The listing builds one solid part. Answer for the finished solid, in the listing's coordinates (mm). A direction names the side the tool comes from. Coordinates: 2 decimals unless noted, no trailing zeros. Order: outer loops, then holes, each group sorted by start corner. A loop starts at its lowest first (then second) coordinate and runs counter-clockwise, first axis right, second up. Notation, with made-up numbers: (45.25, -6) -> (55.25, -6) arc R24 ccw to (55.25, 27) -> close; hole circle Ø6 at (35, 81.5). An arc over 180 degrees is marked (long way). Write each question's results on one line, items separated by ' | '. Start each with the question number.
(1) A tool of negligible diameter and unlimited length cuts with its end or side. For faces 1 (the face through (125, -2, 9.7)), 2 (the face through (273.001, -1.959, 6.783)), 3 (the face through (157, -2, 0)), from which of +Z, -Z, +X, -X, +Y, -Y can it reach the whole face along a straight path? Write none if from no direction.
(2) Determine the mould class of faces 4 (the face through (-22.41, -1.96, 8.88)), 5 (the face through (155, -2, 3)), 6 (the face through (126, 10.564, 11)), 7 (the face through (70.778, -1.959, 3.397)) for opening direction Z: +Z half, -Z half, draft (parallel to the pull), parting line (faces both ways), or undercut.
(3) The part is cut by section A-A, the plane x = 162. Give the vertices of the cut face in (y, z), then the cut area to 3 significant figures.
(4) Straight lines are drawn through the part: L1, parallel to Z at x = 164.5, y = 3.5; L2, parallel to Z at x = 54, y = -12.25; L3, parallel to Z at x = 231, y = -4.75. For each, find the intervals that lie inside material, in ascending order.
(5) The part is cut by section C-C, the plane x = 42. Give the vertices of the cut face in (y, z), then the cut area to 3 significant figures.
(6) The part is cut by section D-D, the plane x = 237. Give the vertices of the cut face in (y, z).
(7) Given pin 1 (12 mm diameter, centred on x = 184.5, y = -3.5, fed in from -Z); pin 2 (1.5 mm diameter, centred on x = 195.5, y = 6.5, fed in from -Z); pin 3 (3 mm diameter, centred on x = 97.47, y = 5.36, fed in from -Z), each flat-ended and moving along its own axis, determine where each tip first touches the part or whether it passes through.
```python
from build123d import *

# Parameters (mm, degrees)
SKETCH1_W                 = 304.8
SKETCH1_H                 = 25.4
BOSS_EXTRUDE2_DEPTH       = 12.7
FILLET1_R                 = 12.7
CUT_EXTRUDE3_DEPTH        = 281.209703849
SKETCH8_W                 = 70
SKETCH8_H                 = 25.4
BOSS_EXTRUDE3_DEPTH       = 9.7
CUT_EXTRUDE4_DEPTH        = 281.209703849
CUT_EXTRUDE5_DEPTH        = 281.209703849
F_6_CLEARANCE_HOLE1_D     = 3.7973
F_6_CLEARANCE_HOLE1_DEPTH = 3


with BuildPart() as part:
    # Sketch1 → Boss-Extrude2 (new body)
    with BuildSketch(Plane.XY):
        with Locations((126.366978193, -2.136448598)):
            Rectangle(SKETCH1_W, SKETCH1_H)
    extrude(amount=BOSS_EXTRUDE2_DEPTH)

    # Fillet1
    fillet1_edges = [part.edges().sort_by_distance(p)[0] for p in [
        (-26.033021807, -2.136448598, 12.7),
        (278.766978193, -2.136448598, 12.7),
    ]]
    fillet(fillet1_edges, radius=FILLET1_R - 0.0001)  # a hair under: the kernel refuses the full size

    # Sketch6 → Cut-Extrude3 (cut, through all)
    with BuildSketch(Plane(origin=(0, 10.563551402, 0), x_dir=(1, 0, 0), z_dir=(0, 1, 0))):
        with BuildLine():
            Line((-23.033021807, 0), (275.766978193, 0))
            ThreePointArc((275.766978193, 0), (272.925913971, -6.858935778), (266.066978193, -9.7))
            Line((266.066978193, -9.7), (-13.333021807, -9.7))
            ThreePointArc((-13.333021807, -9.7), (-20.191957584, -6.858935778), (-23.033021807, 0))
        make_face()
    extrude(amount=-CUT_EXTRUDE3_DEPTH, mode=Mode.SUBTRACT)

    # Sketch8 → Boss-Extrude3 (add)
    with BuildSketch(Plane(origin=(0, 0, 9.7), x_dir=(-1, 0, 0), z_dir=(0, 0, -1))):
        with Locations((-180.266978193, -2.136448598)):
            Rectangle(SKETCH8_W, SKETCH8_H)
        with Locations((-72.466978193, -2.136448598)):
            Rectangle(SKETCH8_W, SKETCH8_H)
    extrude(amount=BOSS_EXTRUDE3_DEPTH)

    # Sketch9 → Cut-Extrude4 (cut, through all)
    with BuildSketch(Plane(origin=(0, 10.563551402, 0), x_dir=(1, 0, 0), z_dir=(0, 1, 0))):
        Polygon((145.266978193, -9.7), (165.266978193, -9.7), (192.266978193, -9.7), (165.266978193, -3), (145.266978193, -3), align=None)
        Polygon((215.266978193, -6.7), (195.266978193, -6.7), (168.266978193, 0), (215.266978193, 0), align=None)
    extrude(amount=-CUT_EXTRUDE4_DEPTH, mode=Mode.SUBTRACT)

    # Sketch12 → Cut-Extrude5 (cut, through all)
    with BuildSketch(Plane(origin=(0, 10.563551402, 0), x_dir=(1, 0, 0), z_dir=(0, 1, 0))):
        Polygon((107.466978193, -9.7), (107.466978193, -3), (87.466978193, -3), (60.466978193, -9.7), align=None)
        Polygon((37.466978193, -6.7), (57.466978193, -6.7), (84.466978193, 0), (37.466978193, 0), align=None)
    extrude(amount=-CUT_EXTRUDE5_DEPTH, mode=Mode.SUBTRACT)

    # #6 Clearance Hole1
    with Locations(Plane.XY.offset(3)):
        with Locations((97.466978193, 5.363551402), (155.266978193, 5.363551402), (155.266978193, -9.636448598), (97.466978193, -9.636448598)):
            Hole(F_6_CLEARANCE_HOLE1_D / 2, depth=F_6_CLEARANCE_HOLE1_DEPTH)


solid = part.part
```
Established:
1) face 1: +Y, -Y | face 2: -Z, +Y, -Y | face 3: -Z, +X, -X, +Y, -Y
2) face 4: +Z half | face 5: undercut | face 6: draft | face 7: -Z half
3) outline: (-14.84, 0) -> (10.56, 0) -> (10.56, 3) -> (-14.84, 3) -> close; (-14.84, 9.7) -> (10.56, 9.7) -> (10.56, 12.7) -> (-14.84, 12.7) -> close | area: 152 mm^2
4) L1: z = 0 to 3, 9.7 to 12.7 | L2: z = 6.7 to 12.7 | L3: z = 9.7 to 12.7
5) outline: (-14.84, 6.7) -> (10.56, 6.7) -> (10.56, 12.7) -> (-14.84, 12.7) -> close | area: 152 mm^2
6) outline: (-14.84, 9.7) -> (10.56, 9.7) -> (10.56, 12.7) -> (-14.84, 12.7) -> close
7) pin 1: stops at z = 2.54 | pin 2: stops at z = 6.57 | pin 3: stops at z = 9.7
